Build history of the part. All positions in model axes, mm. Face numbers are marked on the shaded views. A direction names the side the tool comes from. Coordinates: 2 decimals unless noted, no trailing zeros. Order: outer loops, then holes, each group sorted by start corner. A loop starts at its lowest first (then second) coordinate and runs counter-clockwise, first axis right, second up. Notation, with made-up numbers: M 66,40 L 98,40 A16 ccw 98,46 Z; hole C -35.5,-38.75 d8. An arc over 180 degrees is marked long. Use a Markdown table: item, result. Add a question column.
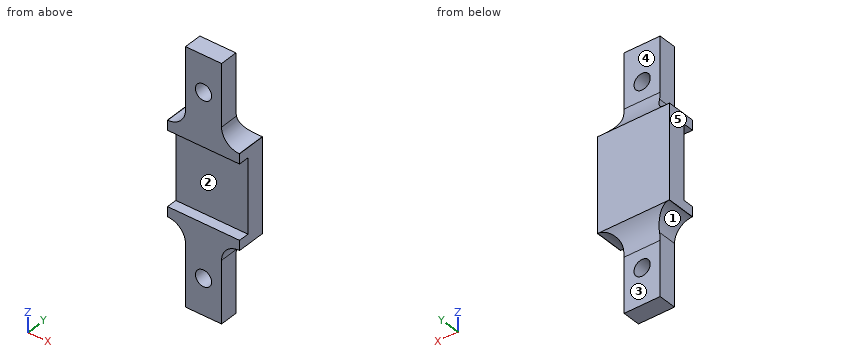
from build123d import *

# Parameters (mm, degrees)
SKETCH009_R          = 2.25
PAD007_DEPTH         = 8
SKETCH010_W          = 20.5
SKETCH010_H          = 2.9
POCKET002_DEPTH      = 20
POCKET003_DEPTH      = 15.001
POCKET003_DEPTH_BACK = 5.001


with BuildPart() as part:
    # Sketch009 → Pad007 (new body)
    with BuildSketch(Plane.XZ):
        with BuildLine():
            Line((40, -13), (40.1, -13))
            ThreePointArc((45, -17.9), (43.564823, -14.435177), (40.1, -13))
            Line((45, -17.9), (45, -35))
            Line((45, -35), (55, -35))
            Line((55, -35), (55, -17.9))
            ThreePointArc((59.9, -13), (56.435177, -14.435177), (55, -17.9))
            Line((59.9, -13), (60, -13))
            Line((60, -13), (60, 13))
            Line((60, 13), (59.9, 13))
            ThreePointArc((55, 17.9), (56.435177, 14.435177), (59.9, 13))
            Line((55, 17.9), (55, 35))
            Line((55, 35), (45, 35))
            Line((45, 35), (45, 17.9))
            ThreePointArc((40.1, 13), (43.564823, 14.435177), (45, 17.9))
            Line((40.1, 13), (40, 13))
            Line((40, 13), (40, -13))
        make_face()
        with Locations((50, -25)):
            Circle(SKETCH009_R, mode=Mode.SUBTRACT)
        with Locations((50, 25)):
            Circle(SKETCH009_R, mode=Mode.SUBTRACT)
    extrude(amount=PAD007_DEPTH)

    # Sketch010 (on Face2 of Pad007) → Pocket002 (cut)
    with BuildSketch(Plane(origin=(40, 0, 0), x_dir=(0, 0, -1), z_dir=(-1, 0, 0))):
        with Locations((0, 6.55)):
            Rectangle(SKETCH010_W, SKETCH010_H)
    extrude(amount=-POCKET002_DEPTH, mode=Mode.SUBTRACT)

    # Sketch011 (on Face13 of Pocket002) → Pocket003 (cut, two sides)
    with BuildSketch(Plane(origin=(45, 0, 0), x_dir=(0, 0, -1), z_dir=(-1, 0, 0))) as pocket003_sk:
        with BuildLine():
            Line((-35, 3), (-19.9, 3))
            ThreePointArc((-13, 0), (-16.138019, 2.217556), (-19.9, 3))
            Line((-35, 0), (-13, 0))
            Line((-35, 3), (-35, 0))
        make_face()
        with BuildLine():
            Line((13, 0), (35, 0))
            Line((35, 0), (35, 3))
            Line((35, 3), (19.9, 3))
            ThreePointArc((19.9, 3), (16.138019, 2.217556), (13, 0))
        make_face()
    extrude(amount=-POCKET003_DEPTH, mode=Mode.SUBTRACT)
    extrude(pocket003_sk.sketch, amount=POCKET003_DEPTH_BACK, mode=Mode.SUBTRACT)


with BuildPart() as part_1:
    # Body005 placement: moved
    add(part.part.moved(Location((0, 19, 0))))


solid = part_1.part
(1) Slice it at B-B on z = 25. Give the cut face in (x, y), and give its area (3 significant figures).
(2) Which spindle directions (+Z, -Z, +X, -X, +Y, -Y) get a long thin tool onto all of the face, cutting with end or side? Do the marked faces 4 and 5. Say none if no direction does.
(3) Mould opens along Z. For the marked faces 1, 2 and 3 say: released by +Z, released by -Z, zero draft, split by the parting line, or undercut.
(4) Slice it at C-C on x = 50. Give the cut face in (y, z) (3 decimals), and give its area (3 significant figures).
(5) Drop flat-ended pins along their axis: P1, Ø11, axis at x = 47.5, z = -26.5, coming from the +Y side; P2, Ø2.5, axis at y = 14.5, z = 28, coming from the -X side; P3, Ø1, axis at y = 18, z = 17.5, coming from the -X side; P4, Ø2, axis at x = 42.5, y = 16, coming from the -Z side. Give the stop position or say it passes through.
(6) Slice it at A-A on y = 12.5. Give the cut face in (x, z), and give its area (3 significant figures).
(7) Drill centre lines: line 1 along Z through (x, y) = (50, 14.25); line 2 along Z through (x, y) = (50, 13.75); line 3 along X through (y, z) = (12.45, 25). Where is each one in solid material? Low to high. Write a range as from..to.
(8) Slice it at D-D on x = 57. Give the cut face in (y, z) (3 decimals).
Solutions:
| question | item | result |
|---|---|---|
| 1 | outline | M 45,11 L 47.75,11 L 47.75,16 L 45,16 Z; M 52.25,11 L 55,11 L 55,16 L 52.25,16 Z |
| 1 | area | 27.5 mm² |
| 2 | face 4 | +Z, +X, -X, +Y |
| 2 | face 5 | +Z, -Z, -X, +Y, -Y |
| 3 | face 1 | released by -Z |
| 3 | face 2 | undercut |
| 3 | face 3 | zero draft |
| 4 | outline | M 11,-35 L 16,-35 L 16,-27.25 L 11,-27.25 Z; M 11,-22.75 L 16,-22.75 L 16,-19.9 A9.435 cw 19,-13 L 19,13 A9.435 cw 16,19.9 L 16,22.75 L 11,22.75 L 11,10.25 L 13.9,10.25 L 13.9,-10.25 L 11,-10.25 Z; M 11,27.25 L 16,27.25 L 16,35 L 11,35 Z |
| 4 | area | 336 mm² |
| 5 | P1 | y = 16 |
| 5 | P2 | x = 45 |
| 5 | P3 | through |
| 5 | P4 | z = -14.37 |
| 6 | outline | M 40,-13 L 40.1,-13 A4.9 cw 45,-17.9 L 45,-35 L 55,-35 L 55,-17.9 A4.9 cw 59.9,-13 L 60,-13 L 60,-10.25 L 40,-10.25 Z; M 40,10.25 L 60,10.25 L 60,13 L 59.9,13 A4.9 cw 55,17.9 L 55,35 L 45,35 L 45,17.9 A4.9 cw 40.1,13 L 40,13 Z; hole C 50,-25 d4.5; hole C 50,25 d4.5 |
| 6 | area | 539 mm² |
| 7 | line 1 | -35..-27.25, -22.75..22.75, 27.25..35 |
| 7 | line 2 | -35..-27.25, -22.75..-10.25, 10.25..22.75, 27.25..35 |
| 7 | line 3 | 45..47.75, 52.25..55 |
| 8 | outline | M 11,-13.95 L 18.112,-13.95 A9.435 cw 19,-13 L 19,13 A9.435 cw 18.112,13.95 L 11,13.95 L 11,10.25 L 13.9,10.25 L 13.9,-10.25 L 11,-10.25 Z |
